Verification items for the finished model (mm, model axes). Round coordinates to 2 decimals unless told otherwise and drop trailing zeros. Order: outer loops, then holes, each group sorted by start corner. A loop starts at its lowest first (then second) coordinate and runs counter-clockwise, first axis right, second up. Notation, with made-up numbers: (76.5, 17.5) -> (107.5, 17.5) arc R18 ccw to (107.5, 40.5) -> close; hole circle Ø6 at (16.5, 71). An arc over 180 degrees is marked (long way). Put each result on its own line as item: value.
from build123d import *

# Parameters (mm, degrees)
SKETCH2_R           = 1.7
BOSS_EXTRUDE1_DEPTH = 7


with BuildPart() as part:
    # Sketch2 → Boss-Extrude1 (new body)
    with BuildSketch(Plane(origin=(0, 0, 0), x_dir=(1, 0, 0), z_dir=(0, 1, 0))):
        with BuildLine():
            Line((21.476765834, 56.323790381), (-17.656175951, 36.537368528))
            ThreePointArc((-17.656175951, 36.537368528), (-20.523911064, 27.803749844), (-11.79029238, 24.93601473))
            Line((-11.79029238, 24.93601473), (30.909707619, 46.52601473))
            ThreePointArc((30.909707619, 46.52601473), (33.5136477, 48.921851075), (34.476765834, 52.326691629))
            Line((34.476765834, 52.326691629), (34.476765834, 79.124442117))
            Line((34.476765834, 79.124442117), (21.476765834, 79.124442117))
            Line((21.476765834, 79.124442117), (21.476765834, 56.323790381))
        make_face()
        with Locations(Location((-14.723234165, 30.736691629, 0), (0, 0, 270))):
            Circle(SKETCH2_R, mode=Mode.SUBTRACT)
        with Locations(Location((27.976765834, 52.326691629, 0), (0, 0, 270))):
            Circle(SKETCH2_R, mode=Mode.SUBTRACT)
    extrude(amount=BOSS_EXTRUDE1_DEPTH)


solid = part.part
Item 1: Gauge pin test, flat ends, axial feed: pin 1 Ø4 at (x, y) = (27.5, 1.5) entering from +Z; pin 2 Ø1 at (x, y) = (-12, 0.5) entering from +Z; pin 3 Ø4 at (x, y) = (11, 5) entering from +Z. Record the tip position at first contact, or that the pin passes through.
Check sheet entries:
pin 1: stops at z = -43.79
pin 2: stops at z = -24.63
pin 3: stops at z = -35.45
Item 2: Release check for a two-part mould opening along Z. For faces 1 (the cylindrical face through (28.487, 3.451, -50.705)), 2 (the flat face through (21.477, 3, -68)), 3 (the cylindrical face through (33.5, 3.5, -48.9)) record: +Z half, -Z half, draft (parallel to the pull), parting line (faces both ways), or undercut.
Check sheet entries:
face 1: undercut
face 2: draft
face 3: +Z half
Item 3: Material ranges on L1, parallel to X at y = 5.75, z = -58; L2, parallel to Z at x = -13.5, y = 6.75; L3, parallel to X at y = 4, z = -53.5, recorded low to high. Write a range as [from, to].
Check sheet entries:
L1: x = [21.48, 34.48]
L2: z = [-38.64, -31.92], [-29.56, -24.35]
L3: x = [15.89, 26.75], [29.21, 34.48]
Item 4: Section check A-A on y = 3.25. Record the boundary of the cut face in (x, z).
Check sheet entries:
outline: (-17.66, -36.54) -> (21.48, -56.32) -> (21.48, -79.12) -> (34.48, -79.12) -> (34.48, -52.33) arc R6.5 ccw to (30.91, -46.53) -> (-11.79, -24.94) arc R6.5 ccw to start; hole circle Ø3.4 at (-14.72, -30.74); hole circle Ø3.4 at (27.98, -52.33)
Item 5: Section check C-C on x = -3.5. Record the boundary of the cut face in (y, z).
Check sheet entries:
outline: (0, -43.7) -> (7, -43.7) -> (7, -29.13) -> (0, -29.13) -> close
Item 6: Section check B-B on z = -69. Record the boundary of the cut face in (x, y), then the cut area to 3 significant figures.
Check sheet entries:
outline: (21.48, 0) -> (34.48, 0) -> (34.48, 7) -> (21.48, 7) -> close
area: 91.0 mm^2
